from build123d import *
from OCP.BRepFilletAPI import BRepFilletAPI_MakeChamfer

# Parameters (mm, degrees)
SKETCH_1_W               = 102
SKETCH_1_H               = 38
EXTRUDE_1_DEPTH          = 5
EXTRUDE_START            = -10
EXTRUDE_2_DEPTH          = 3
SKETCH_23_W              = 92
SKETCH_23_H              = 38
CUT_EXTRUDE_4_DEPTH      = 7
SKETCH_25_W              = 92.5
SKETCH_25_H              = 5
EXTRUDE_3_DEPTH          = 7
SKETCH_21_R              = 1.55
SKETCH_21_R_2            = 5
SKETCH_21_W              = 15
SKETCH_21_H              = 12
CUT_EXTRUDE_1_DEPTH      = 10
CUT_EXTRUDE_7_DEPTH      = 65.08587988
CUT_EXTRUDE_7_DEPTH_BACK = 65.08587988
SKETCH_27_W              = 53
SKETCH_27_H              = 12
CHAMFER_1_SIZE           = 5
CHAMFER_1_SIZE_2         = 10
CHAMFER_2_SIZE           = 5
CHAMFER_2_SIZE_2         = 10
SKETCH2_R                = 1.55
CUT_EXTRUDE1_DEPTH       = 114.710157858
FILLET1_R                = 3
FILLET2_R                = 3


with BuildPart() as part:
    # 草图1 → 凸台-拉伸1 (new, symmetric)
    with BuildSketch(Plane(origin=(0, 0, 0), x_dir=(1, 0, 0), z_dir=(0, 1, 0))):
        Rectangle(SKETCH_1_W, SKETCH_1_H)
    extrude(amount=EXTRUDE_1_DEPTH, both=True)

    # 草图4 → 凸台-拉伸2 (add)
    with BuildSketch(Plane(origin=(0, 5, 0), x_dir=(1, 0, 0), z_dir=(0, 1, 0)).offset(EXTRUDE_START)):
        Polygon((61, -19), (51, -19), (51, 19), (61, 19), (61, 13), (58, 13), (58, -13), (61, -13), align=None)
        Polygon((-61, 19), (-61, 13), (-58, 13), (-58, -13), (-61, -13), (-61, -19), (-51, -19), (-51, 19), align=None)
    extrude(amount=EXTRUDE_2_DEPTH)

    # 草图23 → 切除-拉伸4 (cut)
    with BuildSketch(Plane(origin=(0, 5, 0), x_dir=(1, 0, 0), z_dir=(0, 1, 0))):
        Rectangle(SKETCH_23_W, SKETCH_23_H)
    extrude(amount=-CUT_EXTRUDE_4_DEPTH, mode=Mode.SUBTRACT)

    # 草图25 → 凸台-拉伸3 (add)
    with BuildSketch(Plane(origin=(0, -2, 0), x_dir=(1, 0, 0), z_dir=(0, 1, 0))):
        with Locations((0.25, -8.496322734)):
            Rectangle(SKETCH_25_W, SKETCH_25_H)
        with Locations((0.25, 8.496322734)):
            Rectangle(SKETCH_25_W, SKETCH_25_H)
    extrude(amount=EXTRUDE_3_DEPTH)

    # 草图21 → 切除-拉伸1 (cut)
    with BuildSketch(Plane(origin=(0, -5, 0), x_dir=(-1, 0, 0), z_dir=(0, -1, 0))):
        with Locations(Location((-20, 0, 0), (0, 0, 270))):
            Circle(SKETCH_21_R)
        with Locations(Location((20, 0, 0), (0, 0, 90))):
            Circle(SKETCH_21_R)
        with Locations(Location((0, 0, 0), (0, 0, 90))):
            Circle(SKETCH_21_R_2)
        with Locations((-38.5, 0)):
            Rectangle(SKETCH_21_W, SKETCH_21_H)
        with Locations((38.5, 0)):
            Rectangle(SKETCH_21_W, SKETCH_21_H)
    extrude(amount=-CUT_EXTRUDE_1_DEPTH, mode=Mode.SUBTRACT)

    # 草图27 → 切除-拉伸7 (cut, two sides: drawn at the far end of the back side and taken through both)
    with BuildSketch(Plane.XY.offset(-CUT_EXTRUDE_7_DEPTH_BACK)):
        with Locations((0, 6)):
            Rectangle(SKETCH_27_W, SKETCH_27_H)
    extrude(amount=CUT_EXTRUDE_7_DEPTH + CUT_EXTRUDE_7_DEPTH_BACK, mode=Mode.SUBTRACT)

    # 倒角1
    chamfer_1_edges_1 = [part.edges().sort_by_distance(p)[0] for p in [
        (26.5, 0, -8.496322734),
    ]]
    chamfer_1_side_1 = [part.faces().sort_by_distance(p)[0] for p in [
        (26.5, 0.1, -8.496322734),
    ]]
    chamfer_1_edges_2 = [part.edges().sort_by_distance(p)[0] for p in [
        (26.5, 0, 8.496322734),
    ]]
    chamfer_1_side_2 = [part.faces().sort_by_distance(p)[0] for p in [
        (26.5, 0.1, 8.496322734),
    ]]
    chamfer_1 = BRepFilletAPI_MakeChamfer(part.part.solid().wrapped)
    for e in chamfer_1_edges_1:
        chamfer_1.Add(CHAMFER_1_SIZE - 0.0001, CHAMFER_1_SIZE_2 - 0.0001, e.wrapped, chamfer_1_side_1[0].wrapped)
    for e in chamfer_1_edges_2:
        chamfer_1.Add(CHAMFER_1_SIZE - 0.0001, CHAMFER_1_SIZE_2 - 0.0001, e.wrapped, chamfer_1_side_2[0].wrapped)
    add(Compound.cast(chamfer_1.Shape()), mode=Mode.REPLACE)  # a hair under: the kernel refuses the full size

    # 倒角2
    chamfer_2_edges_1 = [part.edges().sort_by_distance(p)[0] for p in [
        (-26.5, 0, -8.496322734),
    ]]
    chamfer_2_side_1 = [part.faces().sort_by_distance(p)[0] for p in [
        (-26.5, 0.1, -8.496322734),
    ]]
    chamfer_2_edges_2 = [part.edges().sort_by_distance(p)[0] for p in [
        (-26.5, 0, 8.496322734),
    ]]
    chamfer_2_side_2 = [part.faces().sort_by_distance(p)[0] for p in [
        (-26.4, 0, 8.496322734),
    ]]
    chamfer_2 = BRepFilletAPI_MakeChamfer(part.part.solid().wrapped)
    for e in chamfer_2_edges_1:
        chamfer_2.Add(CHAMFER_2_SIZE - 0.0001, CHAMFER_2_SIZE_2 - 0.0001, e.wrapped, chamfer_2_side_1[0].wrapped)
    for e in chamfer_2_edges_2:
        chamfer_2.Add(CHAMFER_2_SIZE_2 - 0.0001, CHAMFER_2_SIZE - 0.0001, e.wrapped, chamfer_2_side_2[0].wrapped)
    add(Compound.cast(chamfer_2.Shape()), mode=Mode.REPLACE)  # a hair under: the kernel refuses the full size

    # Sketch2 → Cut-Extrude1 (cut, through all)
    with BuildSketch(Plane(origin=(51, 0, 0), x_dir=(0, 0, -1), z_dir=(1, 0, 0))):
        with Locations((15, 1.5)):
            Circle(SKETCH2_R)
        with Locations((-15, 1.5)):
            Circle(SKETCH2_R)
    extrude(amount=-CUT_EXTRUDE1_DEPTH, mode=Mode.SUBTRACT)

    # Fillet1
    fillet1_edges = [part.edges().sort_by_distance(p)[0] for p in [
        (-61, -3.5, 19),
        (-61, -3.5, 13),
        (-61, -3.5, -13),
        (-61, -3.5, -19),
        (61, -3.5, -13),
        (61, -3.5, -19),
        (61, -3.5, 19),
        (61, -3.5, 13),
    ]]
    fillet(fillet1_edges, radius=FILLET1_R - 0.0001)  # a hair under: the kernel refuses the full size

    # Fillet2
    fillet2_edges = [part.edges().sort_by_distance(p)[0] for p in [
        (-48.5, 5, -19),
        (-48.5, 5, 19),
        (48.5, 5, 19),
        (48.5, 5, -19),
    ]]
    fillet(fillet2_edges, radius=FILLET2_R)


solid = part.part
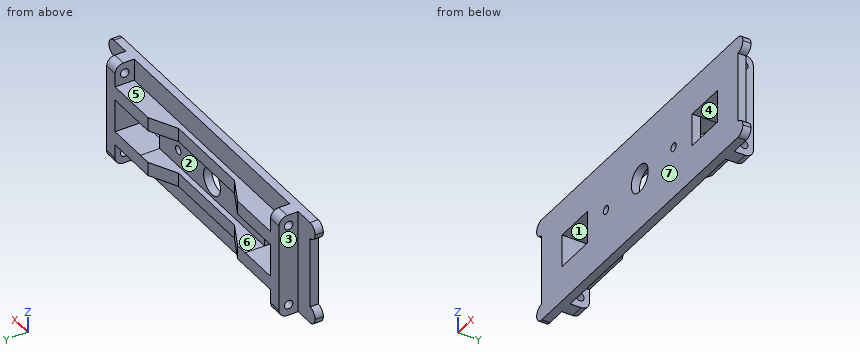
Verification items for the finished model (mm, model axes). Face numbers are marked on the shaded views. A direction names the side the tool comes from. Give positions to 0.01 mm unless a question says otherwise; leave off trailing zeros. Order: outer loops, then holes, each group sorted by start corner. A loop starts at its lowest first (then second) coordinate and runs counter-clockwise, first axis right, second up. Notation, with made-up numbers: M -15,14 L 17,14 A16 cw 17,25 Z; hole C 76,63.5 d1. An arc over 180 degrees is marked long. Answer as a JSON object with one key per item and string values. Group by question number.
1) Scan lines: line 1 along X through (y, z) = (-2.95, 0); line 2 along Z through (x, y) = (31, 2); line 3 along X through (y, z) = (0, 3). Record each from-to range of solid material in increasing order. Write a range as [from, to].
2) Access from +Z, -Z, +X, -X, +Y, -Y to the whole of each face (thin tool, end or side, straight path). Record for the marked faces 1, 2 and 3.
3) Cross-section at D-D (x = 0). Enter the section's corners in (y, z).
4) Cross-section at B-B (x = 29). Enter the section's corners in (y, z).
5) Depth check by flat-ended pin: pin 1 Ø6 at (x, z) = (0, 0) entering from +Y; pin 2 Ø8 at (x, z) = (-58, -4) entering from +Y; pin 3 Ø4 at (y, z) = (1.5, 15) entering from -X; pin 4 Ø4 at (y, z) = (1.5, -15) entering from +X. Enter the tip coordinate at first touch or a pass-through.
6) Mould release check, pull along Z, two halves, no side actions. Record for the marked faces 4, 5, 6 and 7: released by +Z, released by -Z, zero draft, split by the parting line, or undercut.
7) Cross-section at A-A (x = -35.5). Enter the section's corners in (y, z).
Result sheet:
{
 "1": {"line 1": "x = [-58, -46], [-31, -21.55], [-18.45, -5], [5, 18.45], [21.55, 31], [46, 58]", "line 2": "z = [-11, -6], [6, 11]", "line 3": "x = [-51, -46], [46, 51]"},
 "2": {"face 1": "+Y, -Y", "face 2": "+Y", "face 3": "+Z, -Z, -X, +Y"},
 "3": {"outline": "M -5,-19 L -2,-19 L -2,-11 L 0,-11 L 0,-6 L -2,-6 L -2,-5 L -5,-5 Z; M -5,5 L -2,5 L -2,6 L 0,6 L 0,11 L -2,11 L -2,19 L -5,19 Z"},
 "4": {"outline": "M -5,-19 L -2,-19 L -2,-11 L 5,-11 L 5,-6 L -2,-6 L -2,6 L 5,6 L 5,11 L -2,11 L -2,19 L -5,19 Z"},
 "5": {"pin 1": "passes through", "pin 2": "stops at y = -2", "pin 3": "stops at x = -51", "pin 4": "stops at x = 51"},
 "6": {"face 4": "undercut", "face 5": "released by +Z", "face 6": "undercut", "face 7": "zero draft"},
 "7": {"outline": "M -5,-19 L -2,-19 L -2,-11 L 5,-11 L 5,-6 L -5,-6 Z; M -5,6 L 5,6 L 5,11 L -2,11 L -2,19 L -5,19 Z"}
}
